Input: part model. Units: mm. Frame: model coordinates. Face numbers are marked on the shaded views. Round coordinates to 2 decimals unless told otherwise and drop trailing zeros. Order: outer loops, then holes, each group sorted by start corner. A loop starts at its lowest first (then second) coordinate and runs counter-clockwise, first axis right, second up. Notation, with made-up numbers: M 14,30.25 L 21,30.25 A22 cw 21,69.25 Z; hole C 8.25,-26 d1. An arc over 180 degrees is marked long. One line per question, with ' | ' between items.
Autodesk Inventor part; units mm, degrees
ref_plane "YZ Plane" through (0, 0, 0) normal (1, 0, 0) x (0, 1, 0)
ref_plane "XZ Plane" through (0, 0, 0) normal (0, 1, 0) x (-1, 0, 0)
ref_plane "XY Plane" through (0, 0, 0) normal (0, 0, 1) x (1, 0, 0)
sketch "Sketch1" plane through (0, 0, 0) normal (0, 1, 0) x (-1, 0, 0)
  circle A0 centre (0, 0) radius 35
  circle A1 centre (0, 0) radius 34
  circle A2 centre (0, 0) radius 37.5
  circle A3 centre (0, 0) radius 50
  circle A4 centre (0, 0) radius 47.5
  arc A5 (47.6375, -15.1878) -> (47.6375, 15.1878) centre (40, 0) ccw
  arc A6 (15.1878, 47.6375) -> (-15.1878, 47.6375) centre (0, 40) ccw
  arc A7 (-47.6375, 15.1878) -> (-47.6375, -15.1878) centre (-40, 0) ccw
  arc A8 (-15.1878, -47.6375) -> (15.1878, -47.6375) centre (0, -40) ccw
  point P0 (-15.1878, -47.6375)
  point P1 (-47.6375, -15.1878)
  point P2 (-47.6375, 15.1878)
  point P3 (-15.1878, 47.6375)
  point P4 (0, 53)
  point P5 (-53, 0)
  point P6 (-40, 0)
  point P7 (0, -53)
  point P8 (53, 0)
  point P9 (40, 0)
  dimension "d6" = 70
  dimension "d7" = 68
  dimension "d8" = 75
  dimension "d11" = 10
  dimension "d12" = 2.5
  dimension "d13" = 17
  dimension "d14" = 40
  dimension "d17" = 360
  dimension "d27" = 13
  dimension "d30" = 360
extrude "Extrusion1" add sketch "Sketch1" along normal blind 5 contours A2 | A3
extrude "Extrusion2" add sketch "Sketch1" along normal blind 3 contours A4
extrude "Extrusion3" add sketch "Sketch1" along normal blind 4 contours A3 A5 | A3 A6 | A8 A3 | A3 A7
extrude "Extrusion4" add sketch "Sketch1" along normal blind 4 contours A0
hole "Hole1" at (0, 0, 53) at (53, 0, 0) at (0, 0, -53) at (-53, 0, 0) direction (0, 1, 0) diameter 3.242 depth 11.8
sketch "Sketch2" plane through (0, 0, 0) normal (1, 0, 0) x (0, 1, 0)
  line L0 (0, 0) -> (0, 34)
  line L1 (0, 15.1878) -> (0, 47.6375)
  line L2 (0, 34) -> (0, 35)
  line L3 (0, 35) -> (-60, 35)
  line L4 (-60, 35) -> (-60, 5)
  line L5 (-60, 5) -> (0, 34)
  line L6 (-60, 8) -> (-4.1379, 35)
  line L7 (-4.1379, 35) -> (0, 37)
  line L8 (-72, 0) -> (12, 0)
  dimension "d39" = 34
  dimension "d40" = 1
  dimension "d41" = 60
  dimension "d42" = 30
  dimension "d43" = 3
  dimension "d44" = 3
revolve "Revolution1" add sketch "Sketch2" angle 360 about axis through (0, -10, 0) along (0, 1, 0) contours L5 L4 L6 L3 L1
properties part number "LilghtPointLensHolder"
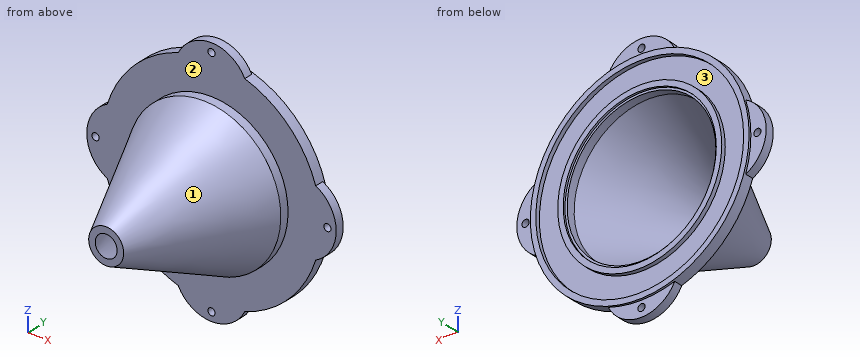
Item 1: Line query: line 1 along Y through (x, z) = (46, -10); line 2 along X through (y, z) = (-21, 6.5); line 3 along X through (y, z) = (-2, -1). Output: solid intervals per line, ascending. Write a range as from..to.
Report:
line 1: 0..3 | line 2: -26.05..-22.95, 22.95..26.05 | line 3: -34.99..-33.02, 33.02..34.99
Item 2: Mould query, pull axis Z, two halves, no side actions, for the marked faces 1, 2 and 3. Classes: +Z half, -Z half, draft (parallel to the pull), parting line (faces both ways), or undercut.
Report:
face 1: parting line | face 2: draft | face 3: undercut
Item 3: First-contact query: pin 1 (5 mm diameter, centred on x = 53, z = 0, fed in from +Y); pin 2 (6 mm diameter, centred on y = -34, z = -2, fed in from +X); pin 3 (10 mm diameter, centred on x = -9.5, z = 25, fed in from +Y). Flat tips, straight axial feed; report the tip coordinate or a pass-through.
Report:
pin 1: y = 4 | pin 2: x = 21.95 | pin 3: y = -4.67
Item 4: Section query C-C, the plane x = 53. Return loops of the section in (y, z).
Report:
outline: M 0,-10.95 L 4,-10.95 L 4,-1.62 L 0,-1.62 Z; M 0,1.62 L 4,1.62 L 4,10.95 L 0,10.95 Z
Item 5: Section query A-A, the plane x = 0. Give the number of separate pieces and of enclosed holes in the cut face, plus the area to 3 significant figures.
Report:
separate pieces: 4 | enclosed holes: 0 | area: 500 mm²
Item 6: Section query B-B, the plane z = -53. Return loops of the section in (x, y).
Report:
outline: M -10.95,0 L -1.62,0 L -1.62,4 L -10.95,4 Z; M 1.62,0 L 10.95,0 L 10.95,4 L 1.62,4 Z
